Part model, mm, in its own coordinate system. A direction names the side the tool comes from. Coordinates: 2 decimals unless noted, no trailing zeros. Loops run counter-clockwise (first coordinate to the right, second up) from the corner with the lowest first, then second, coordinate; pieces in that order, holes last. Notation, with made-up numbers: M 61,43 L 120,43 A22 cw 120,69 Z; hole C 63.5,15 d4. An arc over 180 degrees is marked long. Use a Markdown table: item, result. Add a question column.
1) Pin check, flat tips, straight feed: pin 1 Ø4 at (x, z) = (-5.5, -0.5) entering from -Y; pin 2 Ø4 at (y, z) = (1.5, 0.5) entering from -X; pin 3 Ø2 at (y, z) = (4.5, -1) entering from +X. Stop position of each tip, or through.
2) Tool access for faces 1 (the flat face through (16, 1, 0)), 2 (the flat face through (-1, 5, 0.6)), 3 (the flat face through (-1, 3.2, 0)): list every direction of +Z, -Z, +X, -X, +Y, -Y with a clear straight run to the whole face (end or side of a thin tool).
3) Wall check: probe 1 along Z at (x, y) = (3.5, 2.25); probe 2 along X at (y, z) = (1, 2.75); probe 3 along Y at (x, z) = (8.5, -2). Give the ranges that are in metal, low to high. Write a range as from..to.
4) Pull direction Z, two halves, no side cores. Call faces 4 (the flat face through (-11, 7, -2.4)), 5 (the flat face through (-3, 5, 2.4)), 6 (the flat face through (0, 5, 4)), 7 (the flat face through (-16, 8, 0)): released by +Z, released by -Z, zero draft, split by the parting line, or undercut.
5) Band-saw the part on B-B (z = 2.75). List the corners of the cut face in (x, y), plus the area to 3 significant figures.
Autodesk Inventor part; units mm, degrees
ref_plane "YZ Plane" through (0, 0, 0) normal (1, 0, 0) x (0, 1, 0)
ref_plane "XZ Plane" through (0, 0, 0) normal (0, 1, 0) x (-1, 0, 0)
ref_plane "XY Plane" through (0, 0, 0) normal (0, 0, 1) x (1, 0, 0)
sketch "Sketch2" plane through (0, 0, 0) normal (0, 1, 0) x (-1, 0, 0)
  line L0 (-16, 4) -> (16, 4)
  line L1 (16, 4) -> (16, -4)
  line L2 (16, -4) -> (-16, -4)
  line L3 (-16, -4) -> (-16, 4)
  point P0 (0, 0)
  point P1 (0, 4)
  point P2 (-16, 0)
  dimension "d0" = 32
  dimension "d1" = 8
extrude "Extrusion1" add sketch "Sketch2" along normal blind 9.6
sketch "Sketch10" plane through (0, 0, 0) normal (0, 0, 1) x (1, 0, 0)
  line L0 (-16, 9.6) -> (16, 9.6)
  line L1 (-16, 0) -> (-16, 9.6)
  arc A0 (16, 1.6) -> (-16, 9.6) centre (-16, -58.4) ccw
  line L2 (16, 1.6) -> (16, 9.6)
  line L3 (-16, 0) -> (16, 0)
  line L4 (14.4, 0) -> (14.4, 1.6)
  line L5 (14.4, 1.6) -> (12.4422, 1.6)
  line L6 (-8, 3.2) -> (-8, 7.5163)
  line L7 (-6.4, 7.3024) -> (-6.4, 3.2)
  arc A1 (12.4422, 1.6) -> (-6.4, 7.3024) centre (-16, -58.4) ccw
  arc A2 (-8, 7.5163) -> (-14.4, 7.9807) centre (-16, -58.4) ccw
  line L8 (-14.4, 7.9807) -> (-14.4, 6.4)
  line L9 (1.6, 5.625) -> (1.6, 0)
  line L10 (0, 6.0435) -> (0, 0)
  line L11 (0, 3.2) -> (-6.4, 3.2)
  line L12 (-8, 6.4) -> (-14.4, 6.4)
  line L13 (-14.4, 6.4) -> (-16, 6.4)
  line L14 (16, 0) -> (16, 9.6)
  line L15 (1.6, 0) -> (14.4, 0)
  line L16 (0, 0) -> (-16, 0)
  line L17 (-16, 0) -> (-16, 6.4)
  line L18 (-6.4, 3.2) -> (-8, 3.2)
  dimension "d100" = 1.6
  dimension "d104" = 1.6
  dimension "d105" = 1.6
  dimension "d107" = 1.6
  dimension "d108" = 1.6
  dimension "d113" = 6.4
  dimension "d114" = 3.2
  dimension "d115" = 16
  dimension "d116" = 1.6
extrude "Extrusion7" cut sketch "Sketch10" along normal through all both and the other way through all contours L0 L2 A0 | L13 L12 L6 L18 L11 L10 L3 L1
extrude "Extrusion8" cut sketch "Sketch10" along normal mid plane 4.8 contours L8 A2 L6 L12 | L3 L9 A1 L5 L4 | L11 L7 A1 L10
sketch "Sketch3" plane through (0, 0, 0) normal (0, -1, 0) x (1, 0, 0)
  circle A0 centre (12, 0) radius 2.4 construction
  line L0 (14.4, -2.4) -> (1.6, -2.4)
  line L1 (1.6, -2.4) -> (1.6, 2.4)
  line L2 (1.6, 2.4) -> (14.4, 2.4)
  line L3 (14.4, 2.4) -> (14.4, -2.4)
  line L4 (16, 4) -> (0, 4)
  circle A1 centre (4, 0) radius 2.4 construction
  line L5 (5.3971, 2.4) -> (5.3971, 1.9971)
  line L6 (5.3971, 1.9971) -> (5.9971, 1.3971)
  line L7 (5.9971, 1.3971) -> (6.5971, 1.9971)
  line L8 (6.5971, 1.9971) -> (6.5971, 2.4)
  line L9 (10.6029, 2.4) -> (10.6029, 1.9971)
  line L10 (10.6029, 1.9971) -> (10.0029, 1.3971)
  line L11 (10.0029, 1.3971) -> (9.4029, 1.9971)
  line L12 (9.4029, 1.9971) -> (9.4029, 2.4)
  line L13 (5.3971, -2.4) -> (5.3971, -1.9971)
  line L14 (5.3971, -1.9971) -> (5.9971, -1.3971)
  line L15 (5.9971, -1.3971) -> (6.5971, -1.9971)
  line L16 (6.5971, -1.9971) -> (6.5971, -2.4)
  line L17 (9.4029, -2.4) -> (9.4029, -1.9971)
  line L18 (9.4029, -1.9971) -> (10.0029, -1.3971)
  line L19 (10.0029, -1.3971) -> (10.6029, -1.9971)
  line L20 (10.6029, -1.9971) -> (10.6029, -2.4)
  line L21 (5.6971, 1.6971) -> (4, 0) construction
  dimension "d97" = 4.8
  dimension "d118" = 1.2
extrude "Extrusion2" add sketch "Sketch3" against normal up to next contours L0 L17 L18 L19 L20 | L9 L10 L11 L12 L2 | L0 L13 L14 L15 L16 | L8 L7 L6 L5 L2
sketch "Sketch11" plane through (-8, 3.2, 4) normal (0, -1, 0) x (1, 0, 0)
  line L0 (1.6, -1.6) -> (8, -1.6)
  line L1 (8, -1.6) -> (8, 0)
  line L2 (8, -6.4) -> (1.6, -6.4)
  line L3 (1.6, -6.4) -> (1.6, -1.6)
  circle A0 centre (4, -4) radius 2.4 construction
  line L4 (8, -3.4) -> (6.4, -3.4)
  line L5 (6.4, -3.4) -> (6.4, -4.6)
  line L6 (6.4, -4.6) -> (8, -4.6)
  line L7 (8, -3.4) -> (8, -4.6)
  point P0 (8, -4)
  point P1 (6.4, -4)
  dimension "d119" = 1.2
extrude "Extrusion9" add sketch "Sketch11" against normal up to next
sketch "Sketch12" plane through (-16, 6.4, 4) normal (0, -1, 0) x (1, 0, 0)
  line L0 (1.6, -1.6) -> (8, -1.6)
  line L1 (8, -6.4) -> (1.6, -6.4)
  line L2 (1.6, -6.4) -> (1.6, -1.6)
  line L3 (8, -3.4) -> (6.4, -3.4)
  line L4 (6.4, -3.4) -> (6.4, -4.6)
  line L5 (6.4, -4.6) -> (8, -4.6)
  line L6 (8, -4.6) -> (8, -3.4)
  circle A0 centre (4, -4) radius 2.4 construction
  point P0 (16, -4)
  point P1 (6.4, -4)
  dimension "d122" = 1.2
extrude "Extrusion10" add sketch "Sketch12" against normal up to next
fillet "Fillet1" radius 0.1 8 edges at (-16, 8, 4) (-16, 9.6, 0) (16, 0.8, 4) (16, 0.8, -4) (-16, 8, -4) (0.4924, 7.5697, 4) (0.4924, 7.5697, -4) (16, 1.6, 0)
equation "\"d4\" = lh"
equation "\"d100\" = wall"
equation "\"d104\" = wall"
equation "\"d105\" = 0.333333 * lh - topthk"
equation "\"d107\" = topthk"
equation "\"d108\" = d104"
equation "\"d113\" = 0.666667 * lh"
equation "\"d114\" = 0.333333 * lh"
equation "\"d115\" = 2 * lu"
equation "\"d116\" = wall"
equation "\"d109\" = lu - 2 * wall"
equation "\"d97\" = kd"
equation "\"d22\" = lf"
equation "\"d103\" = d102"
properties part number "11153-Black" material "ABS Plastic"
Entries:
| question | item | result |
|---|---|---|
| 1 | pin 1 | y = 3.2 |
| 1 | pin 2 | x = -8 |
| 1 | pin 3 | x = 12.15 |
| 2 | face 1 | +Z, -Z, +X, +Y, -Y |
| 2 | face 2 | -Y |
| 2 | face 3 | +Z, -Z, -X, -Y |
| 3 | probe 1 | -4..-2.4, 2.4..4 |
| 3 | probe 2 | 0..16 |
| 3 | probe 3 | 3.31..5.03 |
| 4 | face 4 | undercut |
| 4 | face 5 | undercut |
| 4 | face 6 | released by +Z |
| 4 | face 7 | zero draft |
| 5 | outline | M -16,6.4 L -8,6.4 L -8,3.2 L 0,3.2 L 0,0 L 16,0 L 16,1.54 A0.1 ccw 15.95,1.63 A68 ccw -15.9,9.6 A0.1 ccw -16,9.5 Z |
| 5 | area | 147 mm2 |
